Geometry check sheet. Reference: the model listing, model coordinates, mm. A direction names the side the tool comes from. Give positions to 0.01 mm unless a question says otherwise; leave off trailing zeros. Loops run counter-clockwise (first coordinate to the right, second up) from the corner with the lowest first, then second, coordinate; pieces in that order, holes last.
1. Cross-section at A-A, the plane y = 0. Record the cut outline in (x, z).
2. Cross-section at C-C, the plane y = 20. Record the cut outline in (x, z).
3. Release check for a two-part mould opening along Y. For faces 1 (the flat face through (-1.36, 17.61, 0.99)), 2 (the flat face through (-12.12, -17.31, 4.73)), 3 (the flat face through (5.95, 0, 5)) record: +Y half, -Y half, draft (parallel to the pull), parting line (faces both ways), or undercut.
4. Go/stop test with flat-tipped pins: pin 1 Ø1.6 at (x, z) = (7, 5) entering from -Y; pin 2 Ø3 at (x, y) = (-16, -16) entering from +Z; pin 3 Ø1 at (y, z) = (20.5, 1) entering from -X. Record where each tip stops, or that it passes through.
5. Material ranges on L1, parallel to Y at x = 0, z = 3.2; L2, parallel to Y at x = -2.5, z = 1.5; L3, parallel to Z at x = -14, y = -11.5, recorded low to high.
6. Tool access check on faces 4 (the flat face through (-7, 1.5, 5)), 5 (the flat face through (-17.31, 12.12, 4.73)), 6 (the flat face through (7, -1.5, 5)), 7 (the flat face through (2, -20, 2)). Record the directions out of +Z, -Z, +X, -X, +Y, -Y that give a thin tool (end or side, any length) a straight path to the whole face; none if there is none.
7. Cross-section at D-D, the plane x = -5. Record the cut outline in (y, z).
from build123d import *

# Parameters (mm, degrees)
F0_R     = 23
F0_R_2   = 4.05
F1_DEPTH = 3.5
F3_DEPTH = 2.5
F4_W     = 2
F4_H     = 3
F5_DEPTH = 4
F6_R     = 1.5
F7_DEPTH = 25
F9_DEPTH = 2


with BuildPart() as f1:
    # F0 (on Top) → F1 (new body)
    with BuildSketch(Plane.XY):
        Circle(F0_R)
        Circle(F0_R_2, mode=Mode.SUBTRACT)
    extrude(amount=F1_DEPTH)

    # F2 (on face) → F3 (join)
    with BuildSketch(Plane.XY.offset(3.5)):
        with BuildLine():
            Line((16.792617, 11.758317), (17.816557, 12.475287))
            ThreePointArc((17.816557, 12.475287), (15.379572, 15.379572), (12.475287, 17.816557))
            Line((12.475287, 17.816557), (11.758317, 16.792617))
            ThreePointArc((11.758317, 16.792617), (14.495689, 14.495689), (16.792617, 11.758317))
        make_face()
        with BuildLine():
            ThreePointArc((-16.792617, 11.758317), (-14.495689, 14.495689), (-11.758317, 16.792617))
            Line((-11.758317, 16.792617), (-12.475287, 17.816557))
            ThreePointArc((-12.475287, 17.816557), (-15.379572, 15.379572), (-17.816557, 12.475287))
            Line((-17.816557, 12.475287), (-16.792617, 11.758317))
        make_face()
        with BuildLine():
            ThreePointArc((-11.758317, -16.792617), (-14.495689, -14.495689), (-16.792617, -11.758317))
            Line((-16.792617, -11.758317), (-17.816557, -12.475287))
            ThreePointArc((-17.816557, -12.475287), (-15.379572, -15.379572), (-12.475287, -17.816557))
            Line((-12.475287, -17.816557), (-11.758317, -16.792617))
        make_face()
        with BuildLine():
            ThreePointArc((16.792617, -11.758317), (14.495689, -14.495689), (11.758317, -16.792617))
            Line((11.758317, -16.792617), (12.475287, -17.816557))
            ThreePointArc((12.475287, -17.816557), (15.379572, -15.379572), (17.816557, -12.475287))
            Line((17.816557, -12.475287), (16.792617, -11.758317))
        make_face()
    extrude(amount=F3_DEPTH)

    # F4 (on face) → F5 (join)
    with BuildSketch(Plane.XY.offset(3.5)):
        with Locations((6.95, 0)):
            Rectangle(F4_W, F4_H)
        with Locations((-6.95, 0)):
            Rectangle(F4_W, F4_H)
    extrude(amount=F5_DEPTH)

    # F6 (on face) → F7 (cut)
    with BuildSketch(Plane(origin=(0, 0, 0), x_dir=(1, 0, 0), z_dir=(0, 0, -1))):
        with Locations((0, 20)):
            Circle(F6_R)
        with Locations((0, -20)):
            Circle(F6_R)
    extrude(amount=-F7_DEPTH, mode=Mode.SUBTRACT)

    # F8 (on face) → F9 (cut)
    with BuildSketch(Plane(origin=(0, 0, 0), x_dir=(1, 0, 0), z_dir=(0, 0, -1))):
        Polygon((-2.75, 21.587713), (-2.75, 18.412287), (0, 16.824574), (2.75, 18.412287), (2.75, 21.587713), (0, 23.175426), align=None)
        Polygon((2.75, -21.587713), (2.75, -18.412287), (0, -16.824574), (-2.75, -18.412287), (-2.75, -21.587713), (0, -23.175426), align=None)
    extrude(amount=-F9_DEPTH, mode=Mode.SUBTRACT)


solid = f1.part
Result:
1. outline: (-23, 0) - (-4.05, 0) - (-4.05, 3.5) - (-5.95, 3.5) - (-5.95, 7.5) - (-7.95, 7.5) - (-7.95, 3.5) - (-23, 3.5) - close; (4.05, 0) - (23, 0) - (23, 3.5) - (7.95, 3.5) - (7.95, 7.5) - (5.95, 7.5) - (5.95, 3.5) - (4.05, 3.5) - close
2. outline: (-11.36, 0) - (-2.75, 0) - (-2.75, 2) - (-1.5, 2) - (-1.5, 3.5) - (-11.36, 3.5) - close; (1.5, 2) - (2.75, 2) - (2.75, 0) - (11.36, 0) - (11.36, 3.5) - (1.5, 3.5) - close
3. face 1: undercut
3. face 2: -Y half
3. face 3: draft
4. pin 1: stops at y = -1.5
4. pin 2: stops at z = 6
4. pin 3: stops at x = -11.36
5. L1: y = -23 to -21.5, -18.5 to -4.05, 4.05 to 18.5, 21.5 to 23
5. L2: y = -22.86 to -21.73, -18.27 to -3.19, 3.19 to 18.27, 21.73 to 22.86
5. L3: z = 0 to 3.5
6. face 4: +Z, +X, -X, +Y
6. face 5: +Z, -X
6. face 6: +Z, +X, -X, -Y
6. face 7: -Z
7. outline: (-22.45, 0) - (22.45, 0) - (22.45, 3.5) - (-22.45, 3.5) - close
